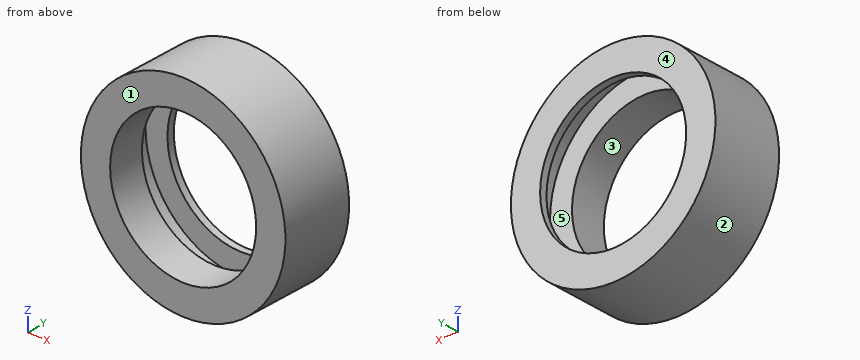
from build123d import *

# Parameters (mm, degrees)
SKETCH3_R          = 7
CUT_EXTRUDE1_DEPTH = 5


with BuildPart() as part:
    # Sketch2 → Revolve1 (revolve)
    with BuildSketch(Plane(origin=(0, 0, 0), x_dir=(0, 0, -1), z_dir=(1, 0, 0))):
        Polygon((5, 3.711600936), (7, 3.711600936), (7, 13.711600936), (5, 13.711600936), (5, 8.211600936), (6.5, 8.211600936), (6.5, 6.211600936), (5, 6.211600936), align=None)
    revolve(axis=Axis((0, 0, 0), (0, 1, 0)))

    # Sketch3 → Cut-Extrude1 (cut)
    with BuildSketch(Plane(origin=(0, 13.711600936, 0), x_dir=(1, 0, 0), z_dir=(0, 1, 0))):
        Circle(SKETCH3_R)
    extrude(amount=-CUT_EXTRUDE1_DEPTH, mode=Mode.SUBTRACT)


solid = part.part
Could you check a few things on this model? Use its own coordinates, in mm. Face numbers are marked on the shaded views. A direction names the side the tool comes from. Round coordinates to 2 decimals unless told otherwise and drop trailing zeros. Loops run counter-clockwise (first coordinate to the right, second up) from the corner with the lowest first, then second, coordinate; pieces in that order, holes last. Notation, with made-up numbers: (31.5, 26.25) - (50.5, 26.25) arc R18 cw to (50.5, 41.25) - close; hole circle Ø8 at (-0.75, 40). An arc over 180 degrees is marked (long way). Write item = value, one per line.
1) If we mould it in two halves opening along X, with no side actions, what happens to the marked faces 1, 2 and 3? For each: pulls with the +X half, pulls with the -X half, needs draft (parallel to the pull), parting line crosses it, or undercut.
Computed:
face_1 = needs draft
face_2 = parting line crosses it
face_3 = undercut
2) I need wall thicknesses on line 1 along Y through (x, z) = (5.25, -1.75); line 2 along X through (y, z) = (4.65, 0); line 3 along Z through (x, y) = (0, 7.55). Which ranges of each line are inside material? Lowest first, please. Write a range as from..to.
Computed:
line_1 = 3.71..6.21, 8.21..8.71
line_2 = -7..-5, 5..7
line_3 = -7..-6.5, 6.5..7
3) Imagine slicing it at A-A (x = 0). Please give me the cut outline in (y, z).
Computed:
outline = (3.71, -7) - (8.71, -7) - (8.71, -5) - (8.21, -5) - (8.21, -6.5) - (6.21, -6.5) - (6.21, -5) - (3.71, -5) - close; (3.71, 5) - (6.21, 5) - (6.21, 6.5) - (8.21, 6.5) - (8.21, 5) - (8.71, 5) - (8.71, 7) - (3.71, 7) - close
4) I'm going to push flat-ended pins straight in: P1, Ø6, axis at x = 0, z = 0, coming from the -Y side; P2, Ø1.5, axis at y = 5.5, z = -5, coming from the +X side; P3, Ø1.5, axis at x = -5.5, y = 4.5, coming from the +Z side; P4, Ø1, axis at x = -2.5, y = 6.5, coming from the -Z side. Where does each tip first touch, or does it pass through?
Computed:
P1 = through
P2 = 5.56
P3 = 5.14
P4 = -6.71
5) Imagine slicing it at D-D (y = 4.15). Please give me the cut outline in (x, z), and give its area (3 significant figures).
Computed:
outline = circle Ø14 at (0, 0); hole circle Ø10 at (0, 0)
area = 75.4 mm2
6) On a 3-axis mill with a long thin cutter (end or side, diameter ignored), from which of +Z, -Z, +X, -X, +Y, -Y can I reach the whole of each face in a straight line? I mean the marked faces 4 and 5. Say none if no direction works.
Computed:
face_4 = +Z, -Z, +X, -X, +Y
face_5 = none
7) Imagine slicing it at B-B (z = 0). Please give me the cut outline in (x, y).
Computed:
outline = (-7, 3.71) - (-5, 3.71) - (-5, 6.21) - (-6.5, 6.21) - (-6.5, 8.21) - (-5, 8.21) - (-5, 8.71) - (-7, 8.71) - close; (5, 3.71) - (7, 3.71) - (7, 8.71) - (5, 8.71) - (5, 8.21) - (6.5, 8.21) - (6.5, 6.21) - (5, 6.21) - close
8) Imagine slicing it at C-C (y = 7.6). Please give me the cut outline in (x, z), and give its area (3 significant figures).
Computed:
outline = circle Ø14 at (0, 0); hole circle Ø13 at (0, 0)
area = 21.2 mm2
